Verification items for the finished model (mm, model axes). Coordinates: 2 decimals unless noted, no trailing zeros. Write each loop counter-clockwise with the first axis right and the second up, starting at its lowest first coordinate (ties: lowest second). Pieces come first, ordered by that corner, then holes. Notation, with made-up numbers: (-38, -18) -> (14, -18) arc R33 cw to (14, 11) -> close; hole circle Ø10 at (35, 72). An arc over 180 degrees is marked (long way). Answer in a Markdown table with one row per item.
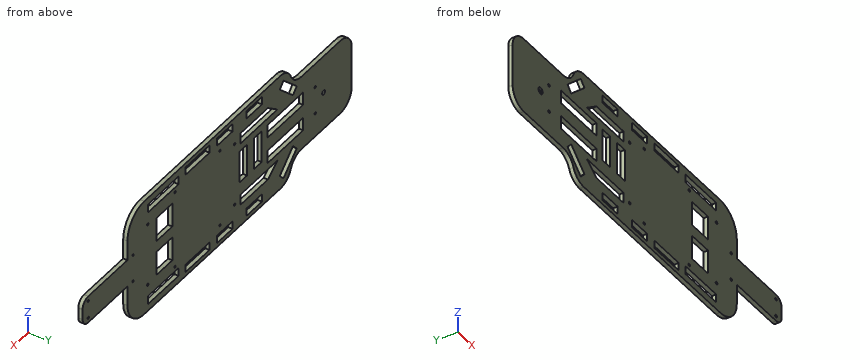
```python
from build123d import *

# Parameters (mm, degrees)
SKETCH1_W                       = 27.36074774
SKETCH1_H                       = 9.31011233
SKETCH1_W_2                     = 63.184924932
SKETCH1_H_2                     = 15.628780018
SKETCH1_W_3                     = 28.563258108
SKETCH1_H_3                     = 28.563258107
SKETCH1_W_4                     = 54.490786644
SKETCH1_H_4                     = 9.808341596
BOSS_EXTRUDE2_DEPTH             = 5
M3X0_5_TAPPED_HOLE1_AT_2_COUNT  = 2
M3X0_5_TAPPED_HOLE1_AT_2_PITCH  = 84.353793631
M3X0_5_TAPPED_HOLE1_AT_3_COUNT  = 2
M3X0_5_TAPPED_HOLE1_AT_3_PITCH  = 80.206374435
M3X0_5_TAPPED_HOLE1_AT_4_COUNT  = 2
M3X0_5_TAPPED_HOLE1_AT_4_PITCH  = 116.569149337
M3X0_5_TAPPED_HOLE1_AT_5_COUNT  = 2
M3X0_5_TAPPED_HOLE1_AT_5_PITCH  = 109.605504319
M3X0_5_TAPPED_HOLE1_AT_6_COUNT  = 2
M3X0_5_TAPPED_HOLE1_AT_6_PITCH  = 241.733079083
M3X0_5_TAPPED_HOLE1_AT_7_COUNT  = 2
M3X0_5_TAPPED_HOLE1_AT_7_PITCH  = 165.040957875
M3X0_5_TAPPED_HOLE1_AT_8_COUNT  = 2
M3X0_5_TAPPED_HOLE1_AT_8_PITCH  = 159.0472187
M3X0_5_TAPPED_HOLE1_AT_9_COUNT  = 2
M3X0_5_TAPPED_HOLE1_AT_9_PITCH  = 237.681260353
M3X0_5_TAPPED_HOLE1_AT_10_COUNT = 2
M3X0_5_TAPPED_HOLE1_AT_10_PITCH = 265.601233698
M3X0_5_TAPPED_HOLE1_AT_11_COUNT = 2
M3X0_5_TAPPED_HOLE1_AT_11_PITCH = 262.61952582
M3X0_5_TAPPED_HOLE1_AT_12_COUNT = 2
M3X0_5_TAPPED_HOLE1_AT_12_PITCH = 405.882449116
M3X0_5_TAPPED_HOLE1_AT_13_COUNT = 2
M3X0_5_TAPPED_HOLE1_AT_13_PITCH = 405.040815845
M3X0_5_TAPPED_HOLE1_AT_14_COUNT = 2
M3X0_5_TAPPED_HOLE1_AT_14_PITCH = 21
SKETCH12_W                      = 13.567630433
SKETCH12_H                      = 38.351630467
SKETCH12_W_2                    = 42.773178661
SKETCH12_H_2                    = 9.31011233
CUT_EXTRUDE1_DEPTH              = 5


with BuildPart() as part:
    # Sketch1 → Boss-Extrude2 (new body)
    with BuildSketch(Plane(origin=(0, 0, 0), x_dir=(1, 0, 0), z_dir=(0, 1, 0))):
        with BuildLine():
            Line((0, -25), (0, 25))
            ThreePointArc((0, 25), (5.857864376, 39.142135624), (20, 45))
            Line((20, 45), (90, 45))
            ThreePointArc((90, 45), (101.180339887, 48.416876048), (108.540496218, 57.5))
            ThreePointArc((108.540496218, 57.5), (115.900652548, 66.583123952), (127.080992435, 70))
            Line((127.080992435, 70), (370, 70))
            ThreePointArc((370, 70), (391.213203436, 61.213203436), (400, 40))
            Line((400, 40), (400, 16.25))
            Line((400, 16.25), (470, 16.25))
            ThreePointArc((470, 16.25), (477.071067812, 13.321067812), (480, 6.25))
            Line((480, 6.25), (480, -6.25))
            ThreePointArc((480, -6.25), (477.071067812, -13.321067812), (470, -16.25))
            Line((470, -16.25), (400, -16.25))
            Line((400, -16.25), (400, -40))
            ThreePointArc((400, -40), (391.213203436, -61.213203436), (370, -70))
            Line((370, -70), (127.080992435, -70))
            ThreePointArc((127.080992435, -70), (115.900652548, -66.583123952), (108.540496218, -57.5))
            ThreePointArc((108.540496218, -57.5), (101.180339887, -48.416876048), (90, -45))
            Line((90, -45), (20, -45))
            ThreePointArc((20, -45), (5.857864376, -39.142135624), (0, -25))
        make_face()
        Polygon((97.973907034, 38.618759958), (121.583872386, 60.672024298), (128.212930651, 53.575032509), (104.602965298, 31.521768169), align=None, mode=Mode.SUBTRACT)
        with Locations((173.68037387, 60.344943835)):
            Rectangle(SKETCH1_W, SKETCH1_H, mode=Mode.SUBTRACT)
        with Locations((226.31962613, 60.344943835)):
            Rectangle(SKETCH1_W, SKETCH1_H, mode=Mode.SUBTRACT)
        Polygon((121.583872386, -60.672024298), (128.212930651, -53.575032509), (104.602965298, -31.521768169), (97.973907034, -38.618759958), align=None, mode=Mode.SUBTRACT)
        with Locations((118.108904399, 15.823440219)):
            Rectangle(SKETCH1_W_2, SKETCH1_H_2, mode=Mode.SUBTRACT)
        with Locations((334.281629054, 21.005470916)):
            Rectangle(SKETCH1_W_3, SKETCH1_H_3, mode=Mode.SUBTRACT)
        with Locations((336.01238987, 56.849636781)):
            Rectangle(SKETCH1_W_4, SKETCH1_H_4, mode=Mode.SUBTRACT)
        with Locations((173.68037387, -60.344943835)):
            Rectangle(SKETCH1_W, SKETCH1_H, mode=Mode.SUBTRACT)
        with Locations((226.31962613, -60.344943835)):
            Rectangle(SKETCH1_W, SKETCH1_H, mode=Mode.SUBTRACT)
        with Locations((336.01238987, -56.849636781)):
            Rectangle(SKETCH1_W_4, SKETCH1_H_4, mode=Mode.SUBTRACT)
        with Locations((334.281629054, -21.005470916)):
            Rectangle(SKETCH1_W_3, SKETCH1_H_3, mode=Mode.SUBTRACT)
        with Locations((118.108904399, -15.823440219)):
            Rectangle(SKETCH1_W_2, SKETCH1_H_2, mode=Mode.SUBTRACT)
    extrude(amount=BOSS_EXTRUDE2_DEPTH)

    # Sketch7 → M3x0.5 Tapped Hole1 (revolve, cut)
    with BuildSketch(Plane(origin=(470, 5, 10.5), x_dir=(0, 0, 1), z_dir=(1, 0, 0))):
        Polygon((0, 0), (0, 5), (1.525, 5), (1.25, 4.725), (1.25, 0), align=None)
    m3x0_5_tapped_hole1 = revolve(axis=Axis((470, 11.35, 10.5), (0, -1, 0)), mode=Mode.SUBTRACT)

    # M3x0.5 Tapped Hole1 at 2: M3x0.5 Tapped Hole1 ×2
    with Locations(*[Vector(-0.9483865106248197, 0, -0.3171167394901739) * (i * M3X0_5_TAPPED_HOLE1_AT_2_PITCH) for i in range(1, M3X0_5_TAPPED_HOLE1_AT_2_COUNT)]):
        add(m3x0_5_tapped_hole1, mode=Mode.SUBTRACT)

    # M3x0.5 Tapped Hole1 at 3: M3x0.5 Tapped Hole1 ×2
    with Locations(*[Vector(-0.9974269571912754, 0, 0.07169006254812285) * (i * M3X0_5_TAPPED_HOLE1_AT_3_PITCH) for i in range(1, M3X0_5_TAPPED_HOLE1_AT_3_COUNT)]):
        add(m3x0_5_tapped_hole1, mode=Mode.SUBTRACT)

    # M3x0.5 Tapped Hole1 at 4: M3x0.5 Tapped Hole1 ×2
    with Locations(*[Vector(-0.9112865611968157, 0, -0.4117727569692806) * (i * M3X0_5_TAPPED_HOLE1_AT_4_PITCH) for i in range(1, M3X0_5_TAPPED_HOLE1_AT_4_COUNT)]):
        add(m3x0_5_tapped_hole1, mode=Mode.SUBTRACT)

    # M3x0.5 Tapped Hole1 at 5: M3x0.5 Tapped Hole1 ×2
    with Locations(*[Vector(-0.9691839830527866, 0, 0.24633799340324214) * (i * M3X0_5_TAPPED_HOLE1_AT_5_PITCH) for i in range(1, M3X0_5_TAPPED_HOLE1_AT_5_COUNT)]):
        add(m3x0_5_tapped_hole1, mode=Mode.SUBTRACT)

    # M3x0.5 Tapped Hole1 at 6: M3x0.5 Tapped Hole1 ×2
    with Locations(*[Vector(-0.972052622294702, 0, -0.23476307096729135) * (i * M3X0_5_TAPPED_HOLE1_AT_6_PITCH) for i in range(1, M3X0_5_TAPPED_HOLE1_AT_6_COUNT)]):
        add(m3x0_5_tapped_hole1, mode=Mode.SUBTRACT)

    # M3x0.5 Tapped Hole1 at 7: M3x0.5 Tapped Hole1 ×2
    with Locations(*[Vector(-0.9390231092578303, 0, -0.34385403920814583) * (i * M3X0_5_TAPPED_HOLE1_AT_7_PITCH) for i in range(1, M3X0_5_TAPPED_HOLE1_AT_7_COUNT)]):
        add(m3x0_5_tapped_hole1, mode=Mode.SUBTRACT)

    # M3x0.5 Tapped Hole1 at 8: M3x0.5 Tapped Hole1 ×2
    with Locations(*[Vector(-0.9744104592657841, 0, 0.22477601489804) * (i * M3X0_5_TAPPED_HOLE1_AT_8_PITCH) for i in range(1, M3X0_5_TAPPED_HOLE1_AT_8_COUNT)]):
        add(m3x0_5_tapped_hole1, mode=Mode.SUBTRACT)

    # M3x0.5 Tapped Hole1 at 9: M3x0.5 Tapped Hole1 ×2
    with Locations(*[Vector(-0.98862347443418, 0, 0.15041152149250553) * (i * M3X0_5_TAPPED_HOLE1_AT_9_PITCH) for i in range(1, M3X0_5_TAPPED_HOLE1_AT_9_COUNT)]):
        add(m3x0_5_tapped_hole1, mode=Mode.SUBTRACT)

    # M3x0.5 Tapped Hole1 at 10: M3x0.5 Tapped Hole1 ×2
    with Locations(*[Vector(-0.9835342087984568, 0, -0.18072205212201886) * (i * M3X0_5_TAPPED_HOLE1_AT_10_PITCH) for i in range(1, M3X0_5_TAPPED_HOLE1_AT_10_COUNT)]):
        add(m3x0_5_tapped_hole1, mode=Mode.SUBTRACT)

    # M3x0.5 Tapped Hole1 at 11: M3x0.5 Tapped Hole1 ×2
    with Locations(*[Vector(-0.994700978251516, 0, 0.10281032956603646) * (i * M3X0_5_TAPPED_HOLE1_AT_11_PITCH) for i in range(1, M3X0_5_TAPPED_HOLE1_AT_11_COUNT)]):
        add(m3x0_5_tapped_hole1, mode=Mode.SUBTRACT)

    # M3x0.5 Tapped Hole1 at 12: M3x0.5 Tapped Hole1 ×2
    with Locations(*[Vector(-0.9978258505204469, 0, -0.0659057814849869) * (i * M3X0_5_TAPPED_HOLE1_AT_12_PITCH) for i in range(1, M3X0_5_TAPPED_HOLE1_AT_12_COUNT)]):
        add(m3x0_5_tapped_hole1, mode=Mode.SUBTRACT)

    # M3x0.5 Tapped Hole1 at 13: M3x0.5 Tapped Hole1 ×2
    with Locations(*[Vector(-0.9998992302925277, 0, 0.014196100183171115) * (i * M3X0_5_TAPPED_HOLE1_AT_13_PITCH) for i in range(1, M3X0_5_TAPPED_HOLE1_AT_13_COUNT)]):
        add(m3x0_5_tapped_hole1, mode=Mode.SUBTRACT)

    # M3x0.5 Tapped Hole1 at 14: M3x0.5 Tapped Hole1 ×2
    with Locations(*[(0, 0, -i * M3X0_5_TAPPED_HOLE1_AT_14_PITCH) for i in range(1, M3X0_5_TAPPED_HOLE1_AT_14_COUNT)]):
        add(m3x0_5_tapped_hole1, mode=Mode.SUBTRACT)

    # Sketch9 → 1/4-20 Tapped Hole1 (revolve, cut)
    with BuildSketch(Plane(origin=(50, 5, 0), x_dir=(0, 0, 1), z_dir=(1, 0, 0))):
        Polygon((0, 0), (0, 5), (3.81, 5), (2.5527, 3.7427), (2.5527, 0), align=None)
    revolve(axis=Axis((50, 11.35, 0), (0, -1, 0)), mode=Mode.SUBTRACT)

    # Sketch12 → Cut-Extrude1 (cut)
    with BuildSketch(Plane(origin=(0, 5, 0), x_dir=(1, 0, 0), z_dir=(0, 1, 0))):
        with Locations((167.418815824, -3.696545403)):
            Rectangle(SKETCH12_W, SKETCH12_H)
        with Locations((193.366452745, -3.696545403)):
            Rectangle(SKETCH12_W, SKETCH12_H)
        with Locations((274.966905924, 60.344943835)):
            Rectangle(SKETCH12_W_2, SKETCH12_H_2)
        with Locations((274.966905924, -60.344943835)):
            Rectangle(SKETCH12_W_2, SKETCH12_H_2)
        Polygon((132.36021003, 31.709406718), (149.471247182, 44.35453871), (198.060388772, 44.35453871), (198.060388772, 31.709406718), align=None)
        Polygon((198.060388772, -31.709406718), (132.36021003, -31.709406718), (149.471247182, -44.35453871), (198.060388772, -44.35453871), align=None)
    extrude(amount=-CUT_EXTRUDE1_DEPTH, mode=Mode.SUBTRACT)


solid = part.part
```
1. Section check C-C, the plane y = 3.25. State how many separate pieces and enclosed holes the cut face has, plus the area to 3 significant figures.
Geometry says:
| item | result |
|---|---|
| separate pieces | 1 |
| enclosed holes | 33 |
| area | 42,900 mm^2 |
2. Depth check by flat-ended pin: P1, Ø2.5, axis at x = 444, y = 3, coming from the +Z side; P2, Ø1.5, axis at y = 3.5, z = -22, coming from the +X side; P3, Ø1.5, axis at y = 4, z = 44, coming from the -X side. Enter the tip coordinate at first touch or a pass-through.
Geometry says:
| item | result |
|---|---|
| P1 | z = 16.25 |
| P2 | x = 400 |
| P3 | x = 11.82 |
3. Thickness scan on line 1 (X direction, y = 2.35, z = 0) (3 decimals); line 2 (Z direction, x = 310, y = 1.85); line 3 (Z direction, x = 286.5, y = 0.6). Record the ranges inside material, lowest first. Write a range as from..to.
Geometry says:
| item | result |
|---|---|
| line 1 | 0..47.447, 52.553..160.635, 174.203..186.583, 200.15..480 |
| line 2 | -70..-61.75, -51.95..51.95, 61.75..70 |
| line 3 | -70..-65, -55.69..55.69, 65..70 |
4. Section check A-A, the plane x = 165.5. Record the boundary of the cut face in (y, z), plus the area to 3 significant figures.
Geometry says:
| item | result |
|---|---|
| outline | (0, -70) -> (5, -70) -> (5, -65) -> (0, -65) -> close; (0, -55.69) -> (5, -55.69) -> (5, -44.35) -> (0, -44.35) -> close; (0, -31.71) -> (5, -31.71) -> (5, -15.48) -> (0, -15.48) -> close; (0, 22.87) -> (5, 22.87) -> (5, 31.71) -> (0, 31.71) -> close; (0, 44.35) -> (5, 44.35) -> (5, 55.69) -> (0, 55.69) -> close; (0, 65) -> (5, 65) -> (5, 70) -> (0, 70) -> close |
| area | 289 mm^2 |
5. Section check B-B, the plane x = 426. Record the boundary of the cut face in (y, z), plus the area to 4 significant figures.
Geometry says:
| item | result |
|---|---|
| outline | (0, -16.25) -> (5, -16.25) -> (5, 16.25) -> (0, 16.25) -> close |
| area | 162.5 mm^2 |
